Input: dimensioned drawing with shaded views. Units: mm. Origin: part minimum x, y, z. Coordinates: 2 decimals unless noted, no trailing zeros. Loops run counter-clockwise (first coordinate to the right, second up) from the corner with the lowest first, then second, coordinate; pieces in that order, holes last.
Item 1: Section query B-B, the plane x = 52. Return the cut outline in (y, z).
Item 2: Section query A-A, the plane z = 18.5. Return the cut outline in (x, y).
Item 3: Line query: probe 1 along Z at (x, y) = (88.5, 43.5). Output: solid intervals per line, ascending.
Item 4: Pin query (flat end, axial travel): pin 1 Ø2 at (x, y) = (35.5, 42.5) entering from +Z; pin 2 Ø12 at (x, z) = (96.5, 12.5) entering from +Y. Return the tip coordinate at first contact, or that it passes through.
Item 5: Section query C-C, the plane y = 14. Return the cut outline in (x, z), then the cut area to 3 significant figures.
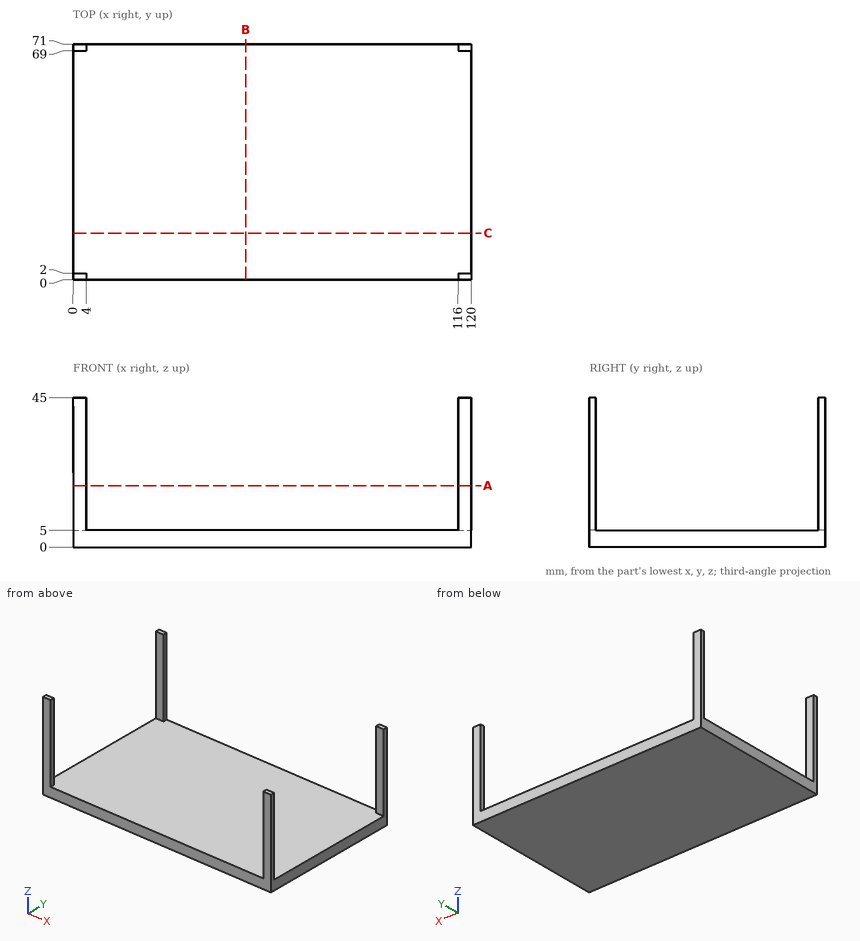
Verdict:
1. outline: (0, 0) - (71, 0) - (71, 5) - (0, 5) - close
2. outline: (0, 0) - (4, 0) - (4, 2) - (0, 2) - close; (0, 69) - (4, 69) - (4, 71) - (0, 71) - close; (116, 0) - (120, 0) - (120, 2) - (116, 2) - close; (116, 69) - (120, 69) - (120, 71) - (116, 71) - close
3. probe 1: z = 0 to 5
4. pin 1: stops at z = 5
4. pin 2: passes through
5. outline: (0, 0) - (120, 0) - (120, 5) - (0, 5) - close
5. area: 600 mm2
